Design review of the part shown in the three views and the two pictorial views. Dimensions are in mm from the part's minimum x, y and z. Coordinates: 2 decimals unless noted, no trailing zeros. Loops run counter-clockwise (first coordinate to the right, second up) from the corner with the lowest first, then second, coordinate; pieces in that order, holes last. Notation, with made-up numbers: (80.25, -38.5) -> (136.25, -38.5) arc R17 ccw to (136.25, -14.5) -> close; hole circle Ø1 at (-17.5, -13). An arc over 180 degrees is marked (long way). One line per item, written item: value.
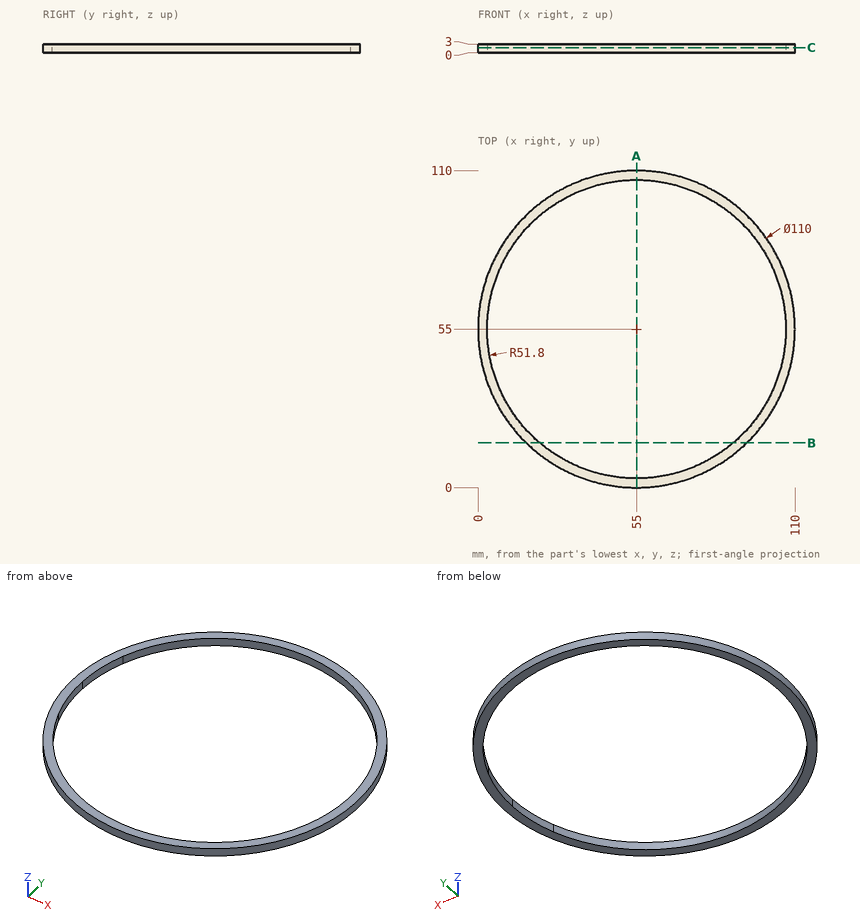
1. Insertion check: pin 1 Ø1 at (x, z) = (15, 1) entering from +Y; pin 2 Ø1.5 at (y, z) = (64.5, 1.5) entering from +X; pin 3 Ø1.5 at (y, z) = (62.5, 2.5) entering from +X. Each pin has a flat end and moves straight along its axis. Give the tip position at first contact, or say it passes through.
Return value:
pin 1: stops at y = 93.27
pin 2: stops at x = 109.3
pin 3: stops at x = 109.58
2. To check wall thickness, follow probe 1 along Y at (x, z) = (54.5, 0.55); probe 2 along Y at (x, z) = (46, 0.4); probe 3 along X at (y, z) = (9.5, 1.4). State the ranges of each line that lie inside material, in increasing order. Write a range as from..to.
Return value:
probe 1: y = 0..3.2, 106.8..110
probe 2: y = 0.74..3.99, 106.01..109.26
probe 3: x = 24.1..30.24, 79.76..85.9
3. Take a section at B-B, the plane y = 15.5. Give the boundary of the cut face in (x, z).
Return value:
outline: (16.73, 0) -> (21.49, 0) -> (21.49, 3) -> (16.73, 3) -> close; (88.51, 0) -> (93.27, 0) -> (93.27, 3) -> (88.51, 3) -> close
4. Take a section at A-A, the plane x = 55. Give the boundary of the cut face in (y, z).
Return value:
outline: (0, 0) -> (3.2, 0) -> (3.2, 3) -> (0, 3) -> close; (106.8, 0) -> (110, 0) -> (110, 3) -> (106.8, 3) -> close
5. Take a section at C-C, the plane z = 1.75. Give the boundary of the cut face in (x, y).
Return value:
outline: circle Ø110 at (55, 55); hole (6.43, 37) arc R51.8 ccw to (103.57, 37) arc R51.8 ccw to (103.57, 73) arc R51.8 ccw to (6.43, 73) arc R51.8 ccw to start
